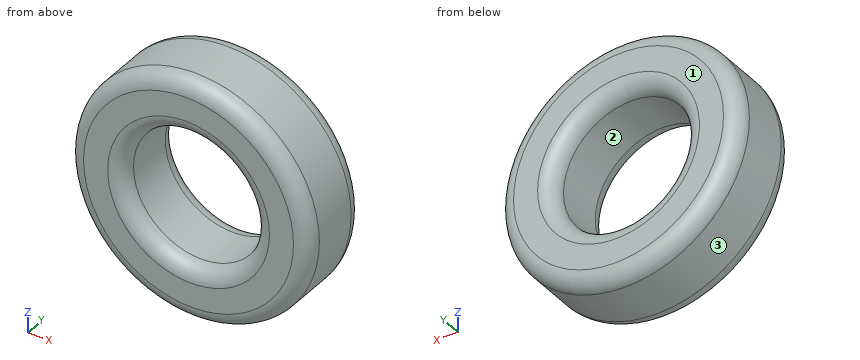
from build123d import *

# Parameters (mm, degrees)
F0_R     = 39.9958807844
F1_DEPTH = 25.4
F2_R     = 21.8277416201
F3_DEPTH = 25.4
F4_R     = 5.08
F5_R     = 5.08


with BuildPart() as f1:
    # F0 (on Front) → F1 (new body)
    with BuildSketch(Plane.XZ):
        Circle(F0_R)
    extrude(amount=F1_DEPTH)

    # F2 (on face) → F3 (cut)
    with BuildSketch(Plane.XZ.offset(25.4)):
        Circle(F2_R)
    extrude(amount=-F3_DEPTH, mode=Mode.SUBTRACT)

    # F4
    f4_edges = [f1.edges().sort_by_distance(p)[0] for p in [
        (-39.995881, -25.4, 0),
        (-21.827742, -25.4, 0),
    ]]
    fillet(f4_edges, radius=F4_R)

    # F5
    f5_edges = [f1.edges().sort_by_distance(p)[0] for p in [
        (-39.995881, 0, 0),
        (-21.827742, 0, 0),
    ]]
    fillet(f5_edges, radius=F5_R)


solid = f1.part
The model under review builds one solid part; all positions refer to its coordinate system, in mm. Face numbers are marked on the shaded views. Round coordinates to 2 decimals unless told otherwise and drop trailing zeros. Loops run counter-clockwise (first coordinate to the right, second up) from the corner with the lowest first, then second, coordinate; pieces in that order, holes last. Notation, with made-up numbers: (7, 8) -> (24, 8) arc R24 ccw to (24, 22) -> close; hole circle Ø6 at (-23, 43). An arc over 180 degrees is marked (long way). Answer as CSV lines item,"result".
1) Add section A-A on z = 0. Write out the cut boundary in (x, y).
Geometry results:
outline,"(-40, -20.32) arc R5.08 ccw to (-34.92, -25.4) -> (-26.91, -25.4) arc R5.08 ccw to (-21.83, -20.32) -> (-21.83, -5.08) arc R5.08 ccw to (-26.91, 0) -> (-34.92, 0) arc R5.08 ccw to (-40, -5.08) -> close; (21.83, -20.32) arc R5.08 ccw to (26.91, -25.4) -> (34.92, -25.4) arc R5.08 ccw to (40, -20.32) -> (40, -5.08) arc R5.08 ccw to (34.92, 0) -> (26.91, 0) arc R5.08 ccw to (21.83, -5.08) -> close"
2) To check wall thickness, follow line 1 along Z through (x, y) = (0, -12); line 2 along Z through (x, y) = (12, -11.5); line 3 along X through (y, z) = (-4.25, -11). State the ranges of each line that lie inside material, in increasing order. Write a range as from..to.
Geometry results:
line 1,"z = -40..-21.83, 21.83..40"
line 2,"z = -38.15..-18.23, 18.23..38.15"
line 3,"x = -38.38..-18.93, 18.93..38.38"
3) For P1, Ø2, axis at y = -18, z = 10.5, coming from the +X side; P2, Ø4, axis at y = -18.5, z = -25, coming from the -X side; P3, Ø12, axis at x = -21, y = -12.5, coming from the +Z side; P4, Ø6, axis at y = -17.5, z = -1, coming from the -X side, all flat-tipped, find the tip position at first contact; note any pin that passes through.
Geometry results:
P1,"stops at x = 38.85"
P2,"stops at x = -32.72"
P3,"stops at z = 37.08"
P4,"stops at x = -40"
4) Add section B-B on x = 0. Write out the cut boundary in (y, z), plus the area to 3 significant figures.
Geometry results:
outline,"(-25.4, -34.92) arc R5.08 ccw to (-20.32, -40) -> (-5.08, -40) arc R5.08 ccw to (0, -34.92) -> (0, -26.91) arc R5.08 ccw to (-5.08, -21.83) -> (-20.32, -21.83) arc R5.08 ccw to (-25.4, -26.91) -> close; (-25.4, 26.91) arc R5.08 ccw to (-20.32, 21.83) -> (-5.08, 21.83) arc R5.08 ccw to (0, 26.91) -> (0, 34.92) arc R5.08 ccw to (-5.08, 40) -> (-20.32, 40) arc R5.08 ccw to (-25.4, 34.92) -> close"
area,"879 mm²"
5) Draft analysis for pull direction X (two halves, no side actions). For the marked faces 1, 2 and 3, state which applies: pulls with the +X half, pulls with the -X half, needs draft (parallel to the pull), parting line crosses it, or undercut.
Geometry results:
face 1,"needs draft"
face 2,"undercut"
face 3,"parting line crosses it"
6) Add section C-C on y = -13.5. Write out the cut boundary in (x, z).
Geometry results:
outline,"circle Ø79.99 at (0, 0); hole circle Ø43.66 at (0, 0)"
7) Add section D-D on y = -22.75. Write out the cut boundary in (x, z).
Geometry results:
outline,"circle Ø78.75 at (0, 0); hole circle Ø44.89 at (0, 0)"
